Design review of the part built by this model. Coordinates are the model's own, in mm. A direction names the side the tool comes from. Coordinates: 2 decimals unless noted, no trailing zeros. Order: outer loops, then holes, each group sorted by start corner. A loop starts at its lowest first (then second) coordinate and runs counter-clockwise, first axis right, second up. Notation, with made-up numbers: (-2, 50.5) -> (4, 50.5) arc R15 cw to (4, 67.5) -> close; hole circle Ø7 at (-30, 29). An arc over 180 degrees is marked (long way). Write item = value, one per line.
```python
from build123d import *

# Parameters (mm, degrees)
EXTRUDE_1_DEPTH     = 20
FILLET_1_R          = 2
SKETCH_2_W          = 7
SKETCH_2_H          = 7
CUT_EXTRUDE_1_DEPTH = 8
CUT_EXTRUDE_4_DEPTH = 29.08914381
CUT_EXTRUDE_5_DEPTH = 29.08914381


with BuildPart() as part:
    # 草图1 → 凸台-拉伸1 (new body)
    with BuildSketch(Plane(origin=(0, 0, 0), x_dir=(0, 0, -1), z_dir=(1, 0, 0))):
        with BuildLine():
            Line((-7, 10), (-7, 0))
            ThreePointArc((-7, 0), (-4.949747468, -4.949747468), (0, -7))
            Line((0, -7), (10, -7))
            Line((10, -7), (10, -10))
            Line((10, -10), (-10, -10))
            Line((-10, -10), (-10, 10))
            Line((-10, 10), (-7, 10))
        make_face()
    extrude(amount=-EXTRUDE_1_DEPTH)

    # 圆角1
    fillet_1_edges = [part.edges().sort_by_distance(p)[0] for p in [
        (-10, -10, 10),
        (-20, -8.5, -10),
        (0, -8.5, -10),
        (-20, 10, 8.5),
        (0, 10, 8.5),
    ]]
    fillet(fillet_1_edges, radius=FILLET_1_R)

    # 草图2 → 切除-拉伸1 (cut, symmetric)
    with BuildSketch(Plane.ZY.offset(10)):
        with Locations((3.5, -3.5)):
            Rectangle(SKETCH_2_W, SKETCH_2_H)
    extrude(amount=CUT_EXTRUDE_1_DEPTH, both=True, mode=Mode.SUBTRACT)

    # 草图3 → 切除-拉伸4 (cut, through all)
    with BuildSketch(Plane(origin=(0, -7, 0), x_dir=(1, 0, 0), z_dir=(0, 1, 0))):
        with BuildLine():
            Line((-12, 4.5), (-12, -1.5))
            ThreePointArc((-12, -1.5), (-10, -3.5), (-8, -1.5))
            Line((-8, -1.5), (-8, 4.5))
            ThreePointArc((-8, 4.5), (-10, 6.5), (-12, 4.5))
        make_face()
    extrude(amount=-CUT_EXTRUDE_4_DEPTH, mode=Mode.SUBTRACT)

    # 草图6 → 切除-拉伸5 (cut, through all)
    with BuildSketch(Plane(origin=(0, 0, 7), x_dir=(-1, 0, 0), z_dir=(0, 0, -1))):
        with BuildLine():
            Line((8, 4.5), (8, -1.5))
            ThreePointArc((8, -1.5), (10, -3.5), (12, -1.5))
            Line((12, -1.5), (12, 4.5))
            ThreePointArc((12, 4.5), (10, 6.5), (8, 4.5))
        make_face()
    extrude(amount=-CUT_EXTRUDE_5_DEPTH, mode=Mode.SUBTRACT)


solid = part.part
```
(1) For L1, parallel to X at y = -8.5, z = 1.5; L2, parallel to Z at x = -16.5, y = 8; L3, parallel to Y at x = -8, z = -8.75, list the stretches that pass through material, from the lowest coordinate up.
Report:
L1 = -20 to -12, -8 to 0
L2 = 7 to 10
L3 = -10 to -7
(2) We need section D-D (z = 7.5). Write out the cut boundary in (x, y), and give its area (3 significant figures).
Report:
outline = (-20, -10) -> (0, -10) -> (0, 8) arc R2 ccw to (-2, 10) -> (-18, 10) arc R2 ccw to (-20, 8) -> close; hole (-12, -1.5) arc R2 ccw to (-8, -1.5) -> (-8, 4.5) arc R2 ccw to (-12, 4.5) -> close
area = 362 mm²
(3) For faces 4 (the cylindrical face through (-10, 6.5, 8.5)), 5 (the flat face through (-2, -6, 6)), 6 (the flat face through (-8, -8, -1)), list the 3-axis set-ups (+Z, -Z, +X, -X, +Y, -Y) from which the entire face can be reached by the end or side of a thin tool; tool diameter is ignored.
Report:
face_4 = +Z, -Z
face_5 = -Z, +Y
face_6 = +Y, -Y
(4) The part is to be moulded in two halves that separate along Z. For faces 1 (the flat face through (0, -6, 5)), 2 (the cylindrical face through (-10, -8.5, 3.5)), 3 (the flat face through (-10, -8, -10)), say which applies: released by +Z, released by -Z, zero draft, split by the parting line, or undercut.
Report:
face_1 = zero draft
face_2 = undercut
face_3 = released by -Z
(5) We need section B-B (z = -1). Write out the cut boundary in (x, y).
Report:
outline = (-20, -10) -> (-12, -10) -> (-12, -7) -> (-20, -7) -> close; (-8, -10) -> (0, -10) -> (0, -7) -> (-8, -7) -> close
(6) We need section A-A (y = 2.75). Write out the cut boundary in (x, z), and give its area (3 significant figures).
Report:
outline = (-20, 7) -> (-12, 7) -> (-12, 10) -> (-20, 10) -> close; (-8, 7) -> (0, 7) -> (0, 10) -> (-8, 10) -> close
area = 48.0 mm²
(7) We need section C-C (x = -12.5). Write out the cut boundary in (y, z), and give its area (3 significant figures).
Report:
outline = (-10, -10) -> (-7, -10) -> (-7, 7) -> (10, 7) -> (10, 10) -> (-8, 10) arc R2 ccw to (-10, 8) -> close
area = 110 mm²
(8) Insertion check: pin 1 (2 mm diameter, centred on y = -2.5, z = 5, fed in from +X); pin 2 (3 mm diameter, centred on x = -6, z = 1, fed in from +Y); pin 3 (1 mm diameter, centred on x = -4, y = -5, fed in from -Z). Each pin has a flat end and moves straight along its axis. Give the tip position at first contact, or say it passes through.
Report:
pin_1 = through
pin_2 = -7
pin_3 = 7
